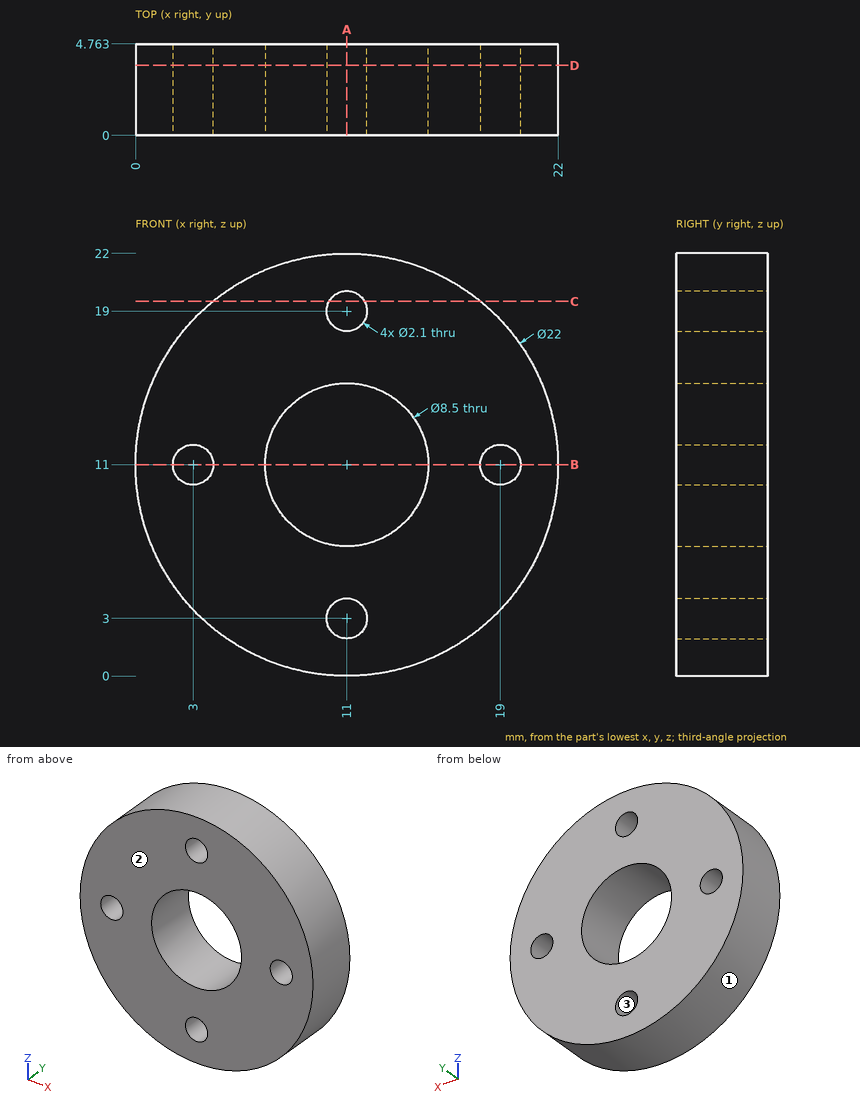
For this review, use the dimensioned drawing (mm, ordinates from the lowest corner) and the shaded views. Coordinates: 2 decimals unless noted, no trailing zeros. Loops run counter-clockwise (first coordinate to the right, second up) from the corner with the lowest first, then second, coordinate; pieces in that order, holes last. Notation, with made-up numbers: (34, -22.75) - (64, -22.75) arc R25 ccw to (64, 13.25) - close; hole circle Ø9 at (31, 53). An arc over 180 degrees is marked (long way). Use one line per item in the form item = value. Start each with the question number.
1) Take a section at A-A (x = 11). State the section outline as (y, z) points.
2) Take a section at D-D (y = 3.65). State the section outline as (x, z) points.
3) To check wall thickness, follow probe 1 along Z at (x, y) = (11, 3); probe 2 along Z at (x, y) = (2.25, 4.5) (1 decimal); probe 3 along X at (y, z) = (2.2, 14.5) (1 decimal). State the ranges of each line that lie inside material, in increasing order. Write a range as from..to.
4) Take a section at B-B (z = 11). State the section outline as (x, y) points.
5) Draft analysis for pull direction X (two halves, no side actions). For the marked faces 1, 2 and 3, state which applies: released by +X, released by -X, zero draft, split by the parting line, or undercut.
6) Take a section at C-C (z = 19.5). State the section outline as (x, y) points.
7) For pin 1 (1.5 mm diameter, centred on x = 15.5, y = 0.5, fed in from -Z); pin 2 (1.5 mm diameter, centred on y = 1.5, z = 15.5, fed in from -X); pin 3 (1 mm diameter, centred on x = 9.5, z = 12, fed in from +Y); pin 4 (2 mm diameter, centred on y = 3.5, z = 13, fed in from +X) (1 decimal), all flat-tipped, find the tip position at first contact; note any pin that passes through.
From the geometry:
q1.outline = (0, 0) - (4.76, 0) - (4.76, 1.95) - (0, 1.95) - close; (0, 4.05) - (4.76, 4.05) - (4.76, 6.75) - (0, 6.75) - close; (0, 15.25) - (4.76, 15.25) - (4.76, 17.95) - (0, 17.95) - close; (0, 20.05) - (4.76, 20.05) - (4.76, 22) - (0, 22) - close
q2.outline = circle Ø22 at (11, 11); hole circle Ø2.1 at (3, 11); hole circle Ø8.5 at (11, 11); hole circle Ø2.1 at (11, 3); hole circle Ø2.1 at (11, 19); hole circle Ø2.1 at (19, 11)
q3.probe_1 = 0..1.95, 4.05..6.75, 15.25..17.95, 20.05..22
q3.probe_2 = 4.3..10.3, 11.7..17.7
q3.probe_3 = 0.6..8.6, 13.4..21.4
q4.outline = (0, 0) - (1.95, 0) - (1.95, 4.76) - (0, 4.76) - close; (4.05, 0) - (6.75, 0) - (6.75, 4.76) - (4.05, 4.76) - close; (15.25, 0) - (17.95, 0) - (17.95, 4.76) - (15.25, 4.76) - close; (20.05, 0) - (22, 0) - (22, 4.76) - (20.05, 4.76) - close
q5.face_1 = split by the parting line
q5.face_2 = zero draft
q5.face_3 = undercut
q6.outline = (4.02, 0) - (10.08, 0) - (10.08, 4.76) - (4.02, 4.76) - close; (11.92, 0) - (17.98, 0) - (17.98, 4.76) - (11.92, 4.76) - close
q7.pin_1 = 0.66
q7.pin_2 = 0.66
q7.pin_3 = through
q7.pin_4 = 22
